Autodesk Inventor part; units mm, degrees
ref_plane "YZ Plane" through (0, 0, 0) normal (1, 0, 0) x (0, 1, 0)
ref_plane "XZ Plane" through (0, 0, 0) normal (0, 1, 0) x (-1, 0, 0)
ref_plane "XY Plane" through (0, 0, 0) normal (0, 0, 1) x (1, 0, 0)
sketch "Sketch1" plane through (0, 0, 0) normal (0, 1, 0) x (-1, 0, 0)
  line L0 (4, 0) -> (18, 0)
  line L1 (22, -4) -> (22, -106)
  line L2 (22, -106) -> (0, -106)
  line L3 (0, -106) -> (0, -4)
  arc A0 (22, -4) -> (18, 0) centre (18, -4) ccw
  arc A1 (4, 0) -> (0, -4) centre (4, -4) ccw
  point P0 (0, 0)
  point P1 (22, 0)
  dimension "d0" = 22
  dimension "d1" = 106
  dimension "d2" = 4
extrude "Extrusion1" add sketch "Sketch1" along normal blind 5
sketch "Sketch2" plane through (0, 5, 0) normal (0, 1, 0) x (1, 0, 0)
  line L0 (-7.75, -15.5804) -> (-7.75, 135.2593) construction
  line L1 (0, 4) -> (0, 106) construction
  line L2 (0, 106) -> (-22, 106)
  point P0 (0, 0)
  point P1 (-7.75, 56.9)
  dimension "d5" = 7.75
  dimension "d6" = 49.1
hole "Hole1" at (-7.75, 5, -56.9) direction (0, -1, 0) diameter 10 end through all
sketch "Sketch3" plane through (0, 5, 0) normal (0, 1, 0) x (1, 0, 0)
  line L0 (-17, -17.788) -> (-17, 124.5417) construction
  line L1 (0, 4) -> (0, 106) construction
  line L2 (0, 106) -> (-22, 106) construction
  line L3 (0, 106) -> (-22, 106) construction
  point P0 (0, 0)
  point P1 (-17, 86)
  point P2 (-17, 21)
  point P3 (-17, 71)
  dimension "d14" = 17
  dimension "d15" = 20
  dimension "d16" = 35
  dimension "d17" = 85
hole "Hole2" at (-17, 5, -86) at (-17, 5, -21) at (-17, 5, -71) direction (0, -1, 0) diameter 3.2 end through all
properties part number "upper plate slide"
The model under review builds one solid part; all positions refer to its coordinate system, in mm. Round coordinates to 2 decimals unless told otherwise and drop trailing zeros. Loops run counter-clockwise (first coordinate to the right, second up) from the corner with the lowest first, then second, coordinate; pieces in that order, holes last. Notation, with made-up numbers: (55, 53.25) -> (101, 53.25) arc R10 ccw to (101, 65.25) -> close; hole circle Ø6 at (-15, 56). An arc over 180 degrees is marked (long way). Answer as CSV lines item,"result".
1) Add section C-C on z = -21. Write out the cut boundary in (x, y).
Geometry results:
outline,"(-22, 0) -> (-18.6, 0) -> (-18.6, 5) -> (-22, 5) -> close; (-15.4, 0) -> (0, 0) -> (0, 5) -> (-15.4, 5) -> close"
2) To check wall thickness, follow line 1 along Z through (x, y) = (-17, 3.5); line 2 along X through (y, z) = (3, -86); line 3 along Z through (x, y) = (-7.75, 3.75). State the ranges of each line that lie inside material, in increasing order. Write a range as from..to.
Geometry results:
line 1,"z = -106..-87.6, -84.4..-72.6, -69.4..-22.6, -19.4..0"
line 2,"x = -22..-18.6, -15.4..0"
line 3,"z = -106..-61.9, -51.9..0"
3) Add section B-B on x = -17. Write out the cut boundary in (y, z), plus the area to 3 significant figures.
Geometry results:
outline,"(0, -106) -> (5, -106) -> (5, -87.6) -> (0, -87.6) -> close; (0, -84.4) -> (5, -84.4) -> (5, -72.6) -> (0, -72.6) -> close; (0, -69.4) -> (5, -69.4) -> (5, -22.6) -> (0, -22.6) -> close; (0, -19.4) -> (5, -19.4) -> (5, 0) -> (0, 0) -> close"
area,"482 mm²"
4) Add section A-A on x = -7.75. Write out the cut boundary in (y, z).
Geometry results:
outline,"(0, -106) -> (5, -106) -> (5, -61.9) -> (0, -61.9) -> close; (0, -51.9) -> (5, -51.9) -> (5, 0) -> (0, 0) -> close"
5) Add section D-D on y = 1.4. Write out the cut boundary in (x, z).
Geometry results:
outline,"(-22, -106) -> (0, -106) -> (0, -4) arc R4 ccw to (-4, 0) -> (-18, 0) arc R4 ccw to (-22, -4) -> close; hole circle Ø3.2 at (-17, -86); hole circle Ø3.2 at (-17, -71); hole circle Ø3.2 at (-17, -21); hole circle Ø10 at (-7.75, -56.9)"
6) Draft analysis for pull direction Z (two halves, no side actions). For faces 1 (the face through (-17.07, 2.46, -87.6)), 2 (the face through (-20.797, 2.465, -1.141)), 3 (the face through (-11, 2, -106)), 4 (the face through (-11, 0, -52)), state which applies: pulls with the +Z half, pulls with the -Z half, needs draft (parallel to the pull), parting line crosses it, or undercut.
Geometry results:
face 1,"undercut"
face 2,"pulls with the +Z half"
face 3,"pulls with the -Z half"
face 4,"needs draft"
7) For P1, Ø8, axis at x = -16.5, z = -49, coming from the -Y side; P2, Ø1.9, axis at x = -17, z = -86, coming from the -Y side, all flat-tipped, find the tip position at first contact; note any pin that passes through.
Geometry results:
P1,"stops at y = 0"
P2,"passes through"
